For this review, take the finished solid that the model builds, in its own axes (mm). Face numbers are marked on the shaded views. A direction names the side the tool comes from. Round coordinates to 2 decimals unless told otherwise and drop trailing zeros. Order: outer loops, then holes, each group sorted by start corner. A loop starts at its lowest first (then second) coordinate and runs counter-clockwise, first axis right, second up. Notation, with made-up numbers: (51, 89) -> (55, 89) arc R15 ccw to (55, 94) -> close; hole circle Ø10 at (36, 16). An arc over 180 degrees is marked (long way). Answer in a Markdown table with one row per item.
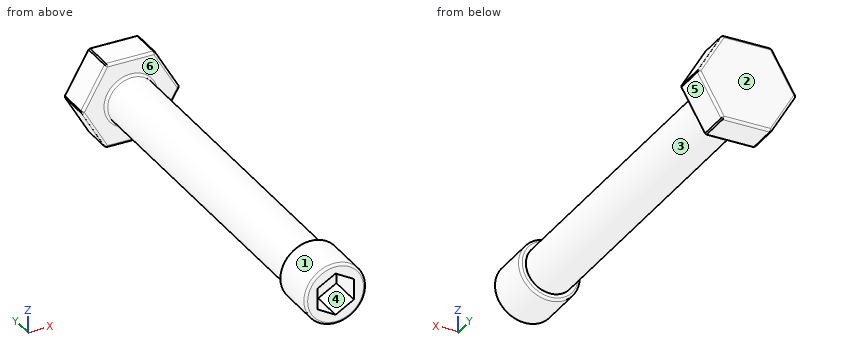
```python
from build123d import *

# Parameters (mm, degrees)
CUT_EXTRUDE2_START = -2.8
SKETCH2_R          = 4.777548175
CUT_EXTRUDE2_DEPTH = 2.8
CUT_EXTRUDE3_DEPTH = 2.7
FILLET1_R          = 0.2


with BuildPart() as part:
    # Sketch1 → Revolve1 (revolve)
    with BuildSketch(Plane.XY):
        Polygon((0, 34.58), (-4, 34.58), (-4, 31.78), (-2, 31.78), (-2, 4), (-2.5, 4), (-2.5, 0), (0, 0), align=None)
    revolve(axis=Axis((0, 37.671641791, 0), (0, -1, 0)))

    # Sketch2 → Cut-Extrude2 (cut)
    with BuildSketch(Plane(origin=(0, 34.58, 0), x_dir=(1, 0, 0), z_dir=(0, 1, 0)).offset(CUT_EXTRUDE2_START)):
        Circle(SKETCH2_R)
        Polygon((-4.041451884, 0), (-2.020725942, -3.5), (2.020725942, -3.5), (4.041451884, 0), (2.020725942, 3.5), (-2.020725942, 3.5), align=None, mode=Mode.SUBTRACT)
    extrude(amount=CUT_EXTRUDE2_DEPTH, mode=Mode.SUBTRACT)

    # Sketch3 → Cut-Extrude3 (cut)
    with BuildSketch(Plane.XZ):
        Polygon((0, 1.732050808), (-1.5, 0.866025404), (-1.5, -0.866025404), (0, -1.732050808), (1.5, -0.866025404), (1.5, 0.866025404), align=None)
    extrude(amount=-CUT_EXTRUDE3_DEPTH, mode=Mode.SUBTRACT)

    # Fillet1
    fillet1_edges = [part.edges().sort_by_distance(p)[0] for p in [
        (4, 31.78, 0),
        (2, 31.78, -3.464101615),
        (-2, 31.78, -3.464101615),
        (-4, 31.78, 0),
        (-2, 31.78, 3.464101615),
        (4, 34.58, 0),
        (2, 34.58, -3.464101615),
        (-2, 34.58, -3.464101615),
        (-4, 34.58, 0),
        (-2, 34.58, 3.464101615),
        (3.031088913, 34.58, -1.75),
        (3.031088913, 34.58, 1.75),
        (0, 34.58, 3.5),
        (-3.031088913, 34.58, 1.75),
        (-3.031088913, 34.58, -1.75),
        (0, 34.58, -3.5),
        (-3.031088913, 31.78, -1.75),
        (-3.031088913, 31.78, 1.75),
        (0, 31.78, 3.5),
        (3.031088913, 31.78, 1.75),
        (3.031088913, 31.78, -1.75),
        (0, 31.78, -3.5),
        (2.5, 0, 0),
        (2.5, 4, 0),
        (2, 31.78, 0),
        (2, 31.78, 3.464101615),
        (2, 34.58, 3.464101615),
    ]]
    fillet(fillet1_edges, radius=FILLET1_R)


solid = part.part
```
Q1. Take a section at A-A, the plane y = 24.5. Write out the cut boundary in (x, z).
Answer key:
| item | result |
|---|---|
| outline | circle Ø4 at (0, 0) |
Q2. Tool access review of the marked faces 4, 5 and 6: name each direction out of +Z, -Z, +X, -X, +Y, -Y from which nothing blocks a thin tool from reaching the whole face with its end or side.
Answer key:
| item | result |
|---|---|
| face 4 | -Y |
| face 5 | -Z, +X, +Y, -Y |
| face 6 | none |
Q3. Clearance check with flat-ended pins moving along their axes: pin 1 Ø1.5 at (x, y) = (0.5, 16) entering from -Z; pin 2 Ø2.5 at (x, z) = (0, 0) entering from -Y; pin 3 Ø1.9 at (y, z) = (0.5, 0) entering from +X. State where each tip first meets the part, or that it passes through.
Answer key:
| item | result |
|---|---|
| pin 1 | stops at z = -2 |
| pin 2 | stops at y = 2.7 |
| pin 3 | stops at x = 2.5 |
Q4. The part is to be moulded in two halves that separate along Y. For the marked faces 1, 2 and 3, say which applies: +Y half, -Y half, draft (parallel to the pull), parting line (faces both ways), or undercut.
Answer key:
| item | result |
|---|---|
| face 1 | draft |
| face 2 | +Y half |
| face 3 | undercut |
Q5. To check wall thickness, follow probe 1 along Y at (x, z) = (3.25, 0.5); probe 2 along Y at (x, z) = (1.25, 2); probe 3 along Y at (x, z) = (0.5, -0.25). State the ranges of each line that lie inside material, in increasing order.
Answer key:
| item | result |
|---|---|
| probe 1 | y = 31.78 to 34.58 |
| probe 2 | y = 0.01 to 3.99, 31.78 to 34.58 |
| probe 3 | y = 2.7 to 34.58 |
